Can you work these out from the model? Positions are in its coordinate system, mm. A direction names the side the tool comes from. Coordinates: 2 decimals unless noted, no trailing zeros. Loops run counter-clockwise (first coordinate to the right, second up) from the corner with the lowest first, then second, coordinate; pieces in that order, holes last. Notation, with made-up numbers: M -1.5,-39.75 L 12.5,-39.75 A30 cw 12.5,-0.75 Z; hole C 61.25,35 d1. An arc over 180 degrees is marked long. Answer as a JSON object with one key per item and string values. Group by question number.
Item 1: Suppose I cut it at A-A (z = 62). Write out the boundary of the cut face in (x, y), then the cut area to 3 significant figures.
Item 2: Suppose I cut it at B-B (y = -8.5). Write out the boundary of the cut face in (x, z), then the cut area to 3 significant figures.
Item 3: We'd pull the mould along X, two halves only. Please class faces 3 (the cylindrical face through (0.51, -2.67, 5.68)), 4 (the cylindrical face through (11.731, -14.493, 121.526)), 5 (the flat face through (15, -8, 62)): +X half, -X half, draft (parallel to the pull), parting line (faces both ways), or undercut.
Item 4: Suppose I cut it at C-C (z = 104). Write out the boundary of the cut face in (x, y), then the cut area to 3 significant figures.
Item 5: Suppose I cut it at D-D (x = 11.25). Count the separate pieces of the cut face and the enclosed holes in it, then the cut area to 3 significant figures.
Item 6: Which directions (+Z, -Z, +X, -X, +Y, -Y) give clear straight access to the entire face, cutting with the end or side of a thin tool? Please do faces 1 (the flat face through (1, -8, 62)), 2 (the flat face through (7, 0, 62)).
Item 7: If I drill on line 1 (X direction, y = -14.7, z = 15); line 2 (Y direction, x = 14.2, z = 27); line 3 (Y direction, x = 11, z = 83.5), over which ranges is the centre line in solid material (lowest first)?
```python
from build123d import *

# Parameters (mm, degrees)
SKETCH_1_W          = 15
SKETCH_1_H          = 15
SKETCH_1_W_2        = 13
SKETCH_1_H_2        = 13
EXTRUDE_1_DEPTH     = 125
SKETCH_2_R          = 1.6
CUT_EXTRUDE_1_DEPTH = 127.787223331
SKETCH_3_R          = 1.6
CUT_EXTRUDE_2_DEPTH = 127.787223331


with BuildPart() as part:
    # 草图1 → 拉伸-薄壁1 (new body)
    with BuildSketch(Plane.XY):
        with Locations((7.5, -7.5)):
            Rectangle(SKETCH_1_W, SKETCH_1_H)
        with Locations((7.5, -7.5)):
            Rectangle(SKETCH_1_W_2, SKETCH_1_H_2, mode=Mode.SUBTRACT)
    extrude(amount=EXTRUDE_1_DEPTH)

    # 草图2 → 切除-拉伸1 (cut, through all)
    with BuildSketch(Plane(origin=(15, 0, 0), x_dir=(0, 0, -1), z_dir=(1, 0, 0))):
        with Locations((-62, -3.75)):
            Circle(SKETCH_2_R)
        with Locations((-62, -11.25)):
            Circle(SKETCH_2_R)
        with Locations((-52, -11.25)):
            Circle(SKETCH_2_R)
        with Locations((-52, -3.75)):
            Circle(SKETCH_2_R)
        with Locations((-17, -3.75)):
            Circle(SKETCH_2_R)
        with Locations((-17, -11.25)):
            Circle(SKETCH_2_R)
        with Locations((-27, -11.25)):
            Circle(SKETCH_2_R)
        with Locations((-27, -3.75)):
            Circle(SKETCH_2_R)
        with Locations((-4.5, -3.75)):
            Circle(SKETCH_2_R)
        with Locations((-4.5, -11.25)):
            Circle(SKETCH_2_R)
    extrude(amount=-CUT_EXTRUDE_1_DEPTH, mode=Mode.SUBTRACT)

    # 草图3 → 切除-拉伸2 (cut, through all)
    with BuildSketch(Plane(origin=(0, 0, 0), x_dir=(1, 0, 0), z_dir=(0, 1, 0))):
        with Locations(Location((3.75, -5, 0), (0, 0, 270))):
            Circle(SKETCH_3_R)
        with Locations(Location((11.25, -5, 0), (0, 0, 90))):
            Circle(SKETCH_3_R)
        with Locations(Location((11.25, -15, 0), (0, 0, 270))):
            Circle(SKETCH_3_R)
        with Locations(Location((3.75, -15, 0), (0, 0, 90))):
            Circle(SKETCH_3_R)
        with Locations(Location((3.75, -57.5, 0), (0, 0, 270))):
            Circle(SKETCH_3_R)
        with Locations(Location((11.25, -57.5, 0), (0, 0, 90))):
            Circle(SKETCH_3_R)
        with Locations(Location((11.25, -67.5, 0), (0, 0, 270))):
            Circle(SKETCH_3_R)
        with Locations(Location((3.75, -67.5, 0), (0, 0, 90))):
            Circle(SKETCH_3_R)
        with Locations(Location((3.75, -110, 0), (0, 0, 270))):
            Circle(SKETCH_3_R)
        with Locations(Location((11.25, -110, 0), (0, 0, 90))):
            Circle(SKETCH_3_R)
        with Locations(Location((11.25, -120, 0), (0, 0, 270))):
            Circle(SKETCH_3_R)
        with Locations(Location((3.75, -120, 0), (0, 0, 90))):
            Circle(SKETCH_3_R)
    extrude(amount=-CUT_EXTRUDE_2_DEPTH, mode=Mode.SUBTRACT)


solid = part.part
```
From the geometry:
{
 "1": {"outline": "M 0,-15 L 15,-15 L 15,-12.85 L 14,-12.85 L 14,-14 L 1,-14 L 1,-12.85 L 0,-12.85 Z; M 0,-9.65 L 1,-9.65 L 1,-5.35 L 0,-5.35 Z; M 0,-2.15 L 1,-2.15 L 1,-1 L 14,-1 L 14,-2.15 L 15,-2.15 L 15,0 L 0,0 Z; M 14,-9.65 L 15,-9.65 L 15,-5.35 L 14,-5.35 Z", "area": "43.2 mm2"},
 "2": {"outline": "M 0,0 L 1,0 L 1,125 L 0,125 Z; M 14,0 L 15,0 L 15,125 L 14,125 Z", "area": "250 mm2"},
 "3": {"face 3": "draft", "face 4": "undercut", "face 5": "+X half"},
 "4": {"outline": "M 0,-15 L 15,-15 L 15,0 L 0,0 Z; hole M 1,-14 L 14,-14 L 14,-1 L 1,-1 Z", "area": "56.0 mm2"},
 "5": {"separate pieces": "14", "enclosed holes": "0", "area": "212 mm2"},
 "6": {"face 1": "+Z, -Z", "face 2": "+Z, -Z, +X, -X, +Y"},
 "7": {"line 1": "0 to 2.15, 5.35 to 9.65, 12.85 to 15", "line 2": "-15 to -12.85, -9.65 to -5.35, -2.15 to 0", "line 3": "-15 to -14, -1 to 0"}
}
